Drawing for the job (mm, zero at the part's lowest x, y, z). A direction names the side the tool comes from. Give positions to 0.01 mm unless a question says otherwise; leave off trailing zeros. Order: outer loops, then holes, each group sorted by start corner. A loop starts at its lowest first (then second) coordinate and runs counter-clockwise, first axis right, second up. Notation, with made-up numbers: (2.5, 36) - (47.5, 36) arc R21 ccw to (47.5, 46) - close; hole circle Ø3 at (70.25, -1.75). An arc over 180 degrees is marked (long way). Use a Markdown table: item, result. Add a question column.
(1) Which spindle directions (+Z, -Z, +X, -X, +Y, -Y) get a long thin tool onto all of the face, cutting with end or side? Do the marked faces 1, 2 and 3. Say none if no direction does.
(2) Slice it at B-B (z = 10). Write the cut outline in (x, y).
(3) Slice it at C-C (x = 28.5). Write the cut outline in (y, z).
(4) Slice it at A-A (x = 11). Write the cut outline in (y, z).
(5) Wall check: line 1 (X direction, y = 13.5, z = 3.5); line 2 (Z direction, x = 25, y = 9.5); line 3 (Z direction, x = 5, y = 11.5). Give the ranges that are in metal, low to high.
(6) Flat gauge pins, fed straight in: pin 1 (2 mm diameter, centred on y = 11.5, z = 9, fed in from +X); pin 2 (3.5 mm diameter, centred on x = 25, z = 3, fed in from -Y); pin 3 (5 mm diameter, centred on x = 24, z = 16.5, fed in from +Y); pin 4 (2 mm diameter, centred on y = 3.5, z = 13, fed in from +X). Where does each tip first touch, or does it go through?
(7) Mould opens along X. For the marked faces 4, 5 and 6 say: +X half, -X half, draft (parallel to the pull), parting line (faces both ways), or undercut.
(8) Slice it at D-D (y = 13.25). Count the separate pieces of the cut face and the enclosed holes in it, then the cut area to 3 significant figures.
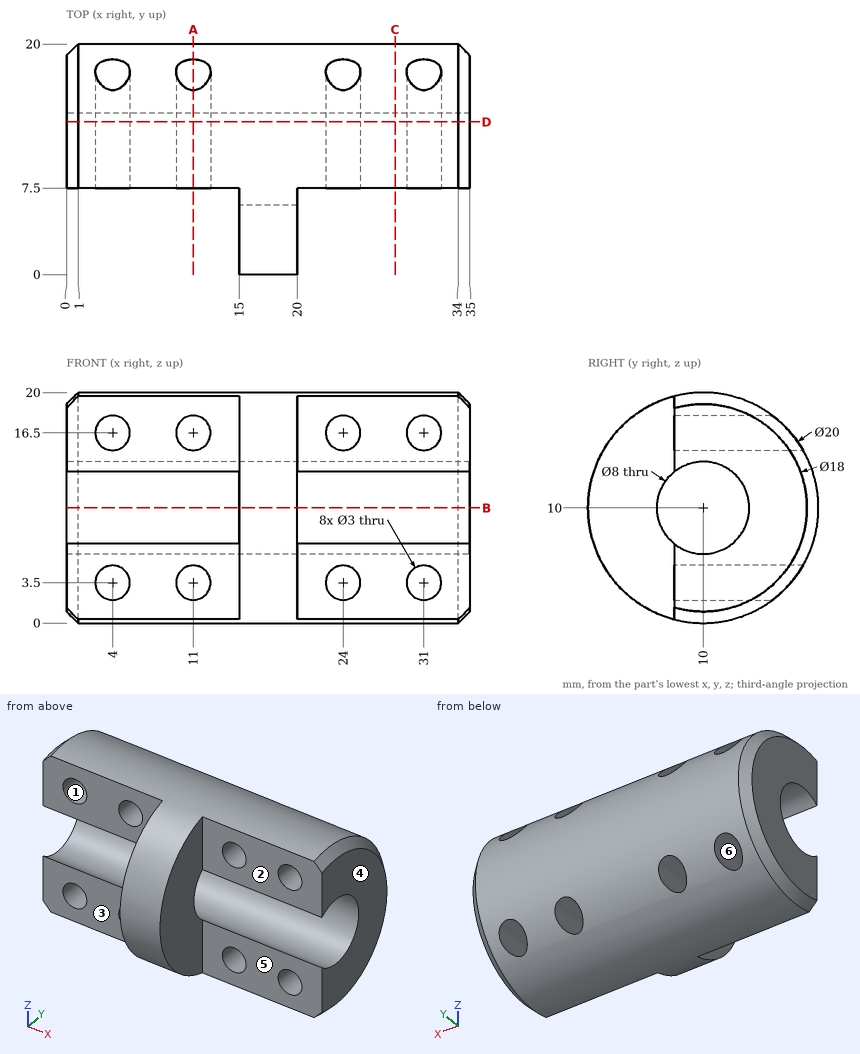
Solution:
| question | item | result |
|---|---|---|
| 1 | face 1 | +Y, -Y |
| 1 | face 2 | +Z, -Z, +X, -Y |
| 1 | face 3 | +Z, -Z, -X, -Y |
| 2 | outline | (0, 14) - (35, 14) - (35, 19) - (34, 20) - (1, 20) - (0, 19) - close; (15, 0) - (20, 0) - (20, 6) - (15, 6) - close |
| 3 | outline | (7.5, 0.32) arc R10 ccw (long way) to (7.5, 19.68) - (7.5, 13.12) arc R4 cw (long way) to (7.5, 6.88) - close |
| 4 | outline | (7.5, 0.32) arc R10 ccw to (16, 2) - (7.5, 2) - close; (7.5, 5) - (18.66, 5) arc R10 ccw to (18.66, 15) - (7.5, 15) - (7.5, 13.12) arc R4 cw (long way) to (7.5, 6.88) - close; (7.5, 18) - (16, 18) arc R10 ccw to (7.5, 19.68) - close |
| 5 | line 1 | 0 to 2.5, 5.5 to 9.5, 12.5 to 22.5, 25.5 to 29.5, 32.5 to 35 |
| 5 | line 2 | 0.01 to 2.38, 4.62 to 6.03, 13.97 to 15.38, 17.62 to 19.99 |
| 5 | line 3 | 0.11 to 2.38, 4.62 to 6.29, 13.71 to 15.38, 17.62 to 19.89 |
| 6 | pin 1 | through |
| 6 | pin 2 | y = 7.5 |
| 6 | pin 3 | y = 19.17 |
| 6 | pin 4 | x = 20 |
| 7 | face 4 | +X half |
| 7 | face 5 | draft |
| 7 | face 6 | undercut |
| 8 | separate pieces | 2 |
| 8 | enclosed holes | 8 |
| 8 | area | 440 mm2 |
